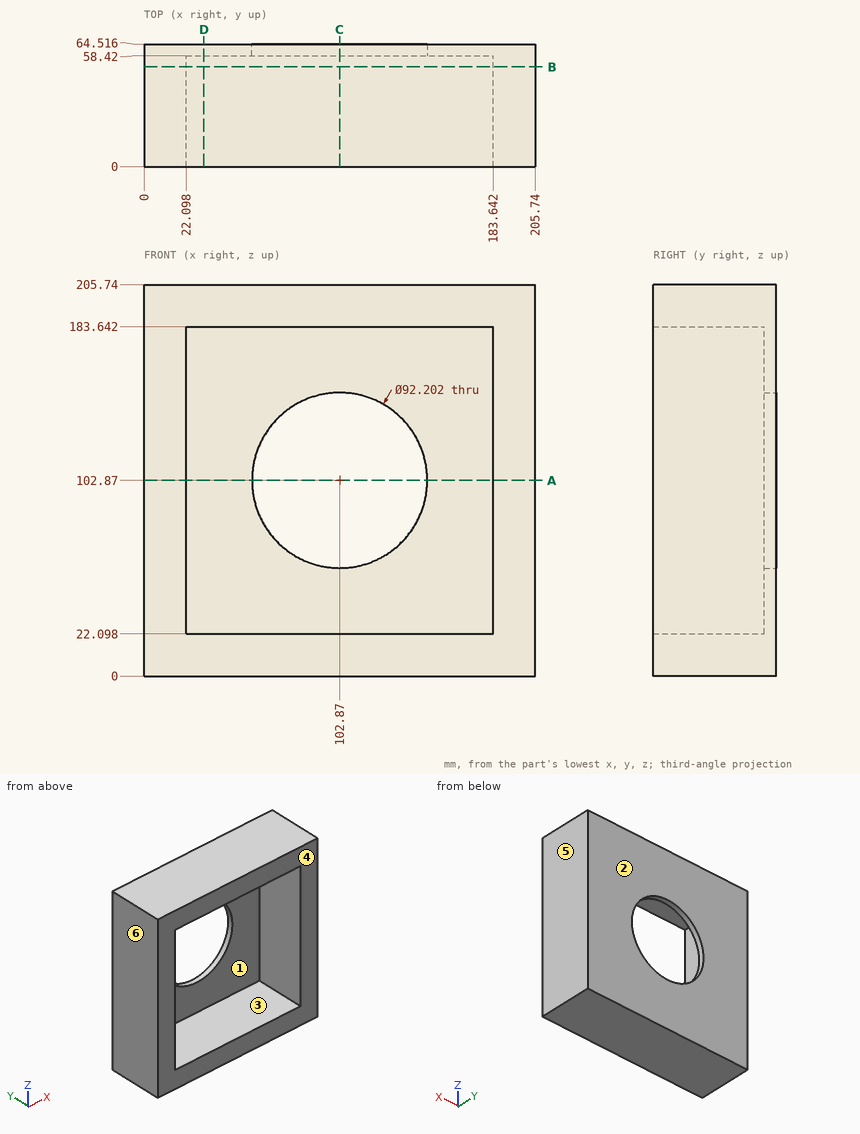
Could you check a few things on this drawing? It's one solid part, dimensions in mm from its lowest x, y, z. A direction names the side the tool comes from. Give positions to 0.01 mm unless a question says otherwise; leave off trailing zeros. Order: outer loops, then holes, each group sorted by start corner. A loop starts at its lowest first (then second) coordinate and runs counter-clockwise, first axis right, second up. Notation, with made-up numbers: M 23,69.25 L 57,69.25 A10 cw 57,88.25 Z; hole C -6.75,-5 d4. An arc over 180 degrees is marked long. Use one line per item in the form item = value. Start each with the question number.
Item 1: If we section it at C-C (x = 102.87): Write out the boundary of the cut face in (y, z), then the cut area to 3 significant figures.
Item 2: Will this pin go through, and if not, where does the flat tip stop? pin 1 Ø12 at (x, z) = (152.5, 138) entering from -Y.
Item 3: If we section it at A-A (z = 102.87): Write out the boundary of the cut face in (x, y).
Item 4: If I drill on line 1 along Z through (x, y) = (102.87, 62); line 2 along X through (y, z) = (29.5, 170), over which ranges is the centre line in solid material (lowest first)?
Item 5: If we section it at D-D (x = 31.5): Write out the boundary of the cut face in (y, z).
Item 6: We'd pull the mould along X, two halves only. Please class the marked faces 3, 4, 5 and 6: +X half, -X half, draft (parallel to the pull), parting line (faces both ways), or undercut.
Item 7: For the marked faces 1 and 2, which set-ups out of +Z, -Z, +X, -X, +Y, -Y let a thin tool reach every point of the face, with its end or its side?
Item 8: If we section it at B-B (y = 52.5): Write out the boundary of the cut face in (x, z), then the cut area to 3 significant figures.
Outcome:
q1.outline = M 0,0 L 64.52,0 L 64.52,56.77 L 58.42,56.77 L 58.42,22.1 L 0,22.1 Z; M 0,183.64 L 58.42,183.64 L 58.42,148.97 L 64.52,148.97 L 64.52,205.74 L 0,205.74 Z
q1.area = 3,270 mm2
q2.pin_1 = 58.42
q3.outline = M 0,0 L 22.1,0 L 22.1,58.42 L 56.77,58.42 L 56.77,64.52 L 0,64.52 Z; M 148.97,58.42 L 183.64,58.42 L 183.64,0 L 205.74,0 L 205.74,64.52 L 148.97,64.52 Z
q4.line_1 = 0 to 56.77, 148.97 to 205.74
q4.line_2 = 0 to 22.1, 183.64 to 205.74
q5.outline = M 0,0 L 64.52,0 L 64.52,205.74 L 0,205.74 L 0,183.64 L 58.42,183.64 L 58.42,22.1 L 0,22.1 Z
q6.face_3 = undercut
q6.face_4 = draft
q6.face_5 = +X half
q6.face_6 = -X half
q7.face_1 = -Y
q7.face_2 = +Z, -Z, +X, -X, +Y
q8.outline = M 0,0 L 205.74,0 L 205.74,205.74 L 0,205.74 Z; hole M 22.1,22.1 L 183.64,22.1 L 183.64,183.64 L 22.1,183.64 Z
q8.area = 16,200 mm2
